Autodesk Fusion 360 part; units mm, degrees
sketch "Sketch1" plane through (0, 0, 0) normal (0, 1, 0) x (1, 0, 0)
  line L0 (36.8758, -36.9029) -> (23.6155, 73.0203)
  circle A0 centre (-1.2046, -43.7212) radius 28
  line L1 (-38.7425, -32.3133) -> (-39.0485, -42.5947)
  circle A1 centre (-1.2046, 74.3196) radius 14
  arc A2 (23.6155, 73.0203) -> (13.7954, 90.0262) centre (-1.2046, 70.0262) ccw
  arc A3 (13.7954, 90.0262) -> (-26.0243, 73.0229) centre (-1.2046, 70.0262) ccw
  line L2 (36.6393, -44.8476) -> (36.8758, -36.9029)
  line L3 (-38.7425, -32.3133) -> (-26.0243, 73.0229)
  arc A4 (-39.0485, -42.5947) -> (36.6393, -44.8476) centre (-1.2046, -43.7212) ccw
  dimension "d1" = 28
  dimension "d2" = 25
  dimension "d3" = 25
  dimension "d4" = 105.3362
extrude "Extrude1" add sketch "Sketch1" along normal blind 0.36
extrude "Extrude2" add 1 faces at (-27.8097, 0, -6.2933) along direction (0, -1, 0) blind 36.4
sketch "Sketch2" plane through (0, 0.36, 0) normal (0, 1, 0) x (-1, 0, 0)
  circle A0 centre (1.2046, -74.3196) radius 14
  circle A1 centre (1.2046, 43.7212) radius 28
  line L0 (38.7425, 32.3133) -> (39.0485, 42.5947)
  arc A2 (39.0485, 42.5947) -> (-36.6393, 44.8476) centre (1.2046, 43.7212) ccw
  line L1 (-36.6393, 44.8476) -> (-36.8758, 36.9029)
  line L2 (-36.8758, 36.9029) -> (-23.6155, -73.0203)
  arc A3 (-23.6155, -73.0203) -> (26.0243, -73.0229) centre (1.2046, -70.0262) ccw
  line L3 (26.0243, -73.0229) -> (38.7425, 32.3133)
  circle A4 centre (0.422, -20.3548) radius 10
  dimension "d9" = 20
extrude "Extrude3" add sketch "Sketch2" along normal blind 20 contours A4
sketch "Sketch3" plane through (0, 20.36, 0) normal (0, 1, 0) x (-1, 0, 0)
  circle A0 centre (0.422, -20.3548) radius 10
  circle A1 centre (0.422, -20.3548) radius 15
  dimension "d12" = 30
extrude "Extrude4" add sketch "Sketch3" along normal blind 10 contours A0 | A1
Check sheet for the modelled part. Datum: model origin and axes. Units: mm. A direction names the side the tool comes from. Round coordinates to 2 decimals unless told otherwise and drop trailing zeros. Loops run counter-clockwise (first coordinate to the right, second up) from the corner with the lowest first, then second, coordinate; pieces in that order, holes last. Notation, with made-up numbers: M 88.5,-12.75 L 131.5,-12.75 A21 cw 131.5,17.25 Z; hole C 34,65.5 d6. An arc over 180 degrees is marked long. One line per question, with ' | ' between items. Start each with the question number.
Item 1: Set-up check for faces 5 (the face through (-8.49, 25.29, -33)), 6 (the face through (30.34, -18.28, -17.29)), 7 (the face through (-10.2, 20.36, -23.5)): record each of +Z, -Z, +X, -X, +Y, -Y from which the full face is reachable in a straight line by a thin tool's end or side.
Item 2: Section check C-C (x = 0). Record the boundary of the cut face in (y, z).
Item 3: Scan lines: probe 1 along Z at (x, y) = (-6.5, -32.5); probe 2 along Z at (x, y) = (-7, -18.5); probe 3 along X at (y, z) = (27.5, -20). Record each from-to range of solid material in increasing order.
Item 4: Gauge pin test, flat ends, axial feed: pin 1 Ø1.5 at (x, y) = (-6.5, -11.5) entering from +Z; pin 2 Ø1.5 at (x, y) = (-5.5, -16.5) entering from +Z; pin 3 Ø6 at (y, z) = (-24.5, 37) entering from -X. Record the tip position at first contact, or that the pin passes through.
Item 5: Section check A-A (x = -20). Record the boundary of the cut face in (y, z).
Item 6: Section check B-B (z = -78). Record the boundary of the cut face in (x, y).
Item 7: Section check D-D (y = -21). Record the boundary of the cut face in (x, z).
Item 8: Release check for a two-part mould opening along X. For faces 1 (the face through (-11.36, -18.28, -92.87)), 2 (the face through (-2, -36.4, -8)), 3 (the face through (-4.24, -18.277, -87.987)), 4 (the face through (13.85, -18.28, 67.33)) record: released by +X, released by -X, zero draft, split by the parting line, or undercut.
Worked out:
1) face 5: +Y | face 6: -Z, +X, +Y, -Y | face 7: none
2) outline: M -36.4,-95 L 0.36,-95 L 0.36,-88.27 L -36.4,-88.27 Z; M -36.4,-60.37 L 0.36,-60.37 L 0.36,-30.35 L 20.36,-30.35 L 20.36,-35.35 L 30.36,-35.35 L 30.36,-5.36 L 20.36,-5.36 L 20.36,-10.36 L 0.36,-10.36 L 0.36,15.75 L -36.4,15.75 Z; M -36.4,71.7 L 0.36,71.7 L 0.36,81.56 L -36.4,81.56 Z
3) probe 1: -94.46 to -87.28, -61.36 to 16.23, 71.22 to 81.21 | probe 2: -94.35 to -87.06, -61.58 to 16.33, 71.11 to 81.14 | probe 3: -15.42 to 14.57
4) pin 1: z = 81.31 | pin 2: z = 81.42 | pin 3: x = -38.97
5) outline: M -36.4,-86.51 L 0.36,-86.51 L 0.36,22.97 L -36.4,22.97 Z; M -36.4,64.48 L 0.36,64.48 L 0.36,76.59 L -36.4,76.59 Z
6) outline: M -24.9,-36.4 L -14.71,-36.4 L -14.71,0.36 L -24.9,0.36 Z; M 12.3,-36.4 L 22.49,-36.4 L 22.49,0.36 L 12.3,0.36 Z
7) outline: M -39.05,42.59 L -38.74,32.31 L -26.02,-73.02 A25 ccw 13.8,-90.03 A25 ccw 23.62,-73.02 L 36.88,36.9 L 36.64,44.85 A37.86 ccw Z; hole C -1.2,43.72 d56; hole C -1.2,-74.32 d28
8) face 1: split by the parting line | face 2: zero draft | face 3: undercut | face 4: undercut
